Geometry: final body of the model. Coordinates: model frame, mm. Coordinates: 2 decimals unless noted, no trailing zeros. Order: outer loops, then holes, each group sorted by start corner. A loop starts at its lowest first (then second) coordinate and runs counter-clockwise, first axis right, second up. Notation, with made-up numbers: M 77,32.5 L 133,32.5 A28 cw 133,62.5 Z; hole C 28,-35 d4. An arc over 180 degrees is marked long. Use CSV: the item, a comma, the result in double quotes. Start each with the question number.
1. Section query C-C on x = -18. Return the cut outline in (y, z).
2. Section query B-B on y = 10. Return the cut outline in (x, z).
3. Section query A-A on x = 10. Return the cut outline in (y, z), and give its area (3 significant figures).
4. Pull-direction query (Y, two-part tool) for faces 1 (the flat face through (0, -13.5, 3)), 2 (the cylindrical face through (-20.747, 0.121, 2.588)), 3 (the flat face through (22, 0, 3)); classes: pulls with the +Y half, pulls with the -Y half, needs draft (parallel to the pull), parting line crosses it, or undercut.
5. Section query D-D on z = 0.8. Return the cut outline in (x, y).
6. First-contact query: P1, Ø2.5, axis at x = -10, y = 10, coming from the -Z side; P2, Ø4, axis at x = 10, y = 10, coming from the +Z side; P3, Ø6.5, axis at x = -18, y = 0, coming from the +Z side. Flat tips, straight axial feed; report the tip coordinate or a pass-through.
7. Material intervals for line 1 (X direction, y = 10, z = 2.75); line 2 (Y direction, x = 10, z = 2.05); line 3 (X direction, y = -0.5, z = 5.55), sorted ascending.
from build123d import *

# Parameters (mm, degrees)
SKETCH1_W                     = 44
SKETCH1_H                     = 27
SKETCH1_R                     = 2.75
BOSS_EXTRUDE1_DEPTH           = 6
CSK_FOR_M3_SFHCS1_D           = 3.4
CSK_FOR_M3_SFHCS1_CSINK_D     = 6.72
CSK_FOR_M3_SFHCS1_CSINK_ANGLE = 90
CHAMFER1_SIZE                 = 0.75


with BuildPart() as part:
    # Sketch1 → Boss-Extrude1 (new body)
    with BuildSketch(Plane.XY):
        Rectangle(SKETCH1_W, SKETCH1_H)
        with Locations((-18, 0)):
            Circle(SKETCH1_R, mode=Mode.SUBTRACT)
        with Locations((18, 0)):
            Circle(SKETCH1_R, mode=Mode.SUBTRACT)
    extrude(amount=BOSS_EXTRUDE1_DEPTH)

    # CSK for M3 SFHCS1 (through all)
    with Locations(Plane.XY.offset(6)):
        with Locations((-10, 10), (10, 10), (10, -10), (-10, -10)):
            CounterSinkHole(CSK_FOR_M3_SFHCS1_D / 2, CSK_FOR_M3_SFHCS1_CSINK_D / 2, counter_sink_angle=CSK_FOR_M3_SFHCS1_CSINK_ANGLE)

    # Chamfer1
    chamfer1_edges = [part.edges().sort_by_distance(p)[0] for p in [
        (-20.75, 0, 6),
        (15.25, 0, 6),
    ]]
    chamfer(chamfer1_edges, length=CHAMFER1_SIZE)


solid = part.part
Results list:
1,outline,"M -13.5,0 L -2.75,0 L -2.75,5.25 L -3.5,6 L -13.5,6 Z; M 2.75,0 L 13.5,0 L 13.5,6 L 3.5,6 L 2.75,5.25 Z"
2,outline,"M -22,0 L -11.7,0 L -11.7,4.34 L -13.36,6 L -22,6 Z; M -8.3,0 L 8.3,0 L 8.3,4.34 L 6.64,6 L -6.64,6 L -8.3,4.34 Z; M 11.7,0 L 22,0 L 22,6 L 13.36,6 L 11.7,4.34 Z"
3,outline,"M -13.5,0 L -11.7,0 L -11.7,4.34 L -13.36,6 L -13.5,6 Z; M -8.3,0 L 8.3,0 L 8.3,4.34 L 6.64,6 L -6.64,6 L -8.3,4.34 Z; M 11.7,0 L 13.5,0 L 13.5,6 L 13.36,6 L 11.7,4.34 Z"
3,area,"116 mm²"
4,face 1,"pulls with the -Y half"
4,face 2,"undercut"
4,face 3,"needs draft"
5,outline,"M -22,-13.5 L 22,-13.5 L 22,13.5 L -22,13.5 Z; hole C -18,0 d5.5; hole C -10,-10 d3.4; hole C -10,10 d3.4; hole C 10,-10 d3.4; hole C 10,10 d3.4; hole C 18,0 d5.5"
6,P1,"passes through"
6,P2,"stops at z = 4.64"
6,P3,"stops at z = 5.75"
7,line 1,"x = -22 to -11.7, -8.3 to 8.3, 11.7 to 22"
7,line 2,"y = -13.5 to -11.7, -8.3 to 8.3, 11.7 to 13.5"
7,line 3,"x = -22 to -21.01, -14.99 to 14.99, 21.01 to 22"
